Read the model definition and answer for the solid it produces. Units are mm, in the model's axes. Face numbers are marked on the shaded views. A direction names the side the tool comes from. Give positions to 0.01 mm unless a question says otherwise; leave off trailing zeros. Loops run counter-clockwise (first coordinate to the right, second up) from the corner with the lowest first, then second, coordinate; pieces in that order, holes last. Notation, with made-up numbers: (-27, -22.75) - (21, -22.75) arc R6 cw to (21, -12.75) - close; hole circle Ø1 at (65.25, -2.5). An arc over 180 degrees is marked (long way). Write each question's results on one line, items separated by ' | '. Start each with the question number.
Q1. The part is cut by section B-B, the plane x = 27.5. Write down the section's boundary in (y, z).
Q2. The part is cut by section A-A, the plane y = 10. State how many separate pieces and enclosed holes the cut face has, plus the area to 3 significant figures.
Q3. For the marked faces 1, 2 and 3, determine the directions among +Z, -Z, +X, -X, +Y, -Y from which every point of the face is accessible in a straight line to the end or side of a thin tool.
Q4. The part is cut by section D-D, the plane x = 8. Write down the section's boundary in (y, z), plus the area to 3 significant figures.
Q5. Given pin 1 (3 mm diameter, centred on x = 11.5, y = 45, fed in from -Z); pin 2 (7 mm diameter, centred on y = 51.5, z = -20, fed in from -X); pin 3 (4.5 mm diameter, centred on y = 60.5, z = 8, fed in from -X), each flat-ended and moving along its own axis, determine where each tip first touches the part or whether it passes through.
Q6. The part is cut by section C-C, the plane y = 53. Write down the section's boundary in (x, z), plus the area to 3 significant figures.
Q7. Find the intervals of material crossed by line 1 (Y direction, x = 50, z = -10); line 2 (X direction, y = 7.5, z = 18.5); line 3 (Z direction, x = 27, y = 11), in increasing order. Write a range as from..to.
Q8. Determine the mould class of the marked faces 4, 5, 6 and 7 for opening direction Z: +Z half, -Z half, draft (parallel to the pull), parting line (faces both ways), or undercut.
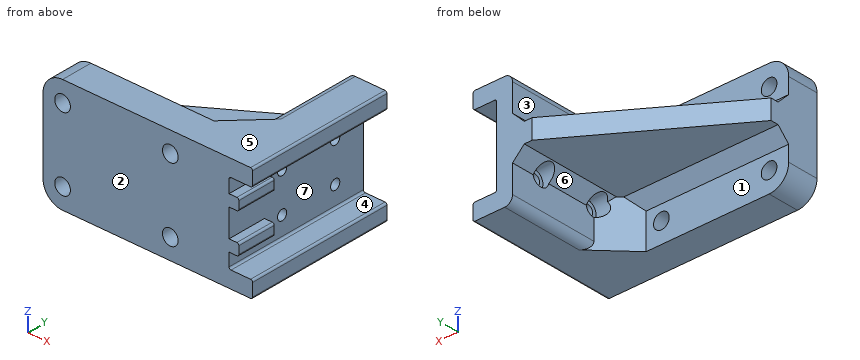
```python
from build123d import *

# Parameters (mm, degrees)
ESQUISSE1_W             = 75
ESQUISSE1_H             = 58
ESQUISSE1_R             = 4
BOSS_EXTRU_1_DEPTH      = 16
ESQUISSE2_W             = 58
ESQUISSE2_H             = 16
BOSS_EXTRU_2_DEPTH      = 20
ESQUISSE3_W             = 8.190465892
ESQUISSE3_H             = 58
BOSS_EXTRU_3_DEPTH      = 60
ESQUISSE4_W             = 8.5
ESQUISSE4_H             = 76
BOSS_EXTRU_4_DEPTH      = 12
ESQUISSE5_W             = 5.9
ESQUISSE5_H             = 20
BOSS_EXTRU_5_DEPTH      = 5
ESQUISSE6_W             = 10
ESQUISSE6_H             = 60
BOSS_EXTRU_6_DEPTH      = 86.809534108
ESQUISSE7_R             = 2.6
ENL_V_MAT_EXTRU_1_DEPTH = 119.965941395
ESQUISSE8_R             = 4.5
ENL_V_MAT_EXTRU_2_DEPTH = 3
ENL_V_MAT_EXTRU_3_DEPTH = 109.45390726
CHANFREIN1_SIZE         = 14
CHANFREIN2_SIZE         = 6
CHANFREIN3_SIZE         = 6
CONG_1_R                = 10
CONG_2_R                = 4
CONG_3_R                = 1
CONG_4_R                = 1


with BuildPart() as part:
    # Esquisse1 → Boss.-Extru.1 (new body)
    with BuildSketch(Plane(origin=(0, 0, 0), x_dir=(1, 0, 0), z_dir=(0, 1, 0))):
        Rectangle(ESQUISSE1_W, ESQUISSE1_H)
        with Locations(Location((-27.5, 18.5, 0), (0, 0, 270))):
            Circle(ESQUISSE1_R, mode=Mode.SUBTRACT)
        with Locations(Location((27.5, 18.5, 0), (0, 0, 90))):
            Circle(ESQUISSE1_R, mode=Mode.SUBTRACT)
        with Locations(Location((27.5, -18.5, 0), (0, 0, 270))):
            Circle(ESQUISSE1_R, mode=Mode.SUBTRACT)
        with Locations(Location((-27.5, -18.5, 0), (0, 0, 90))):
            Circle(ESQUISSE1_R, mode=Mode.SUBTRACT)
    extrude(amount=BOSS_EXTRU_1_DEPTH)

    # Esquisse2 → Boss.-Extru.2 (add)
    with BuildSketch(Plane(origin=(37.5, 0, 0), x_dir=(0, 0, -1), z_dir=(1, 0, 0))):
        with Locations((0, 8)):
            Rectangle(ESQUISSE2_W, ESQUISSE2_H)
    extrude(amount=BOSS_EXTRU_2_DEPTH)

    # Esquisse3 → Boss.-Extru.3 (add)
    with BuildSketch(Plane(origin=(0, 16, 0), x_dir=(1, 0, 0), z_dir=(0, 1, 0))):
        with Locations((53.404767054, 0)):
            Rectangle(ESQUISSE3_W, ESQUISSE3_H)
    extrude(amount=BOSS_EXTRU_3_DEPTH)

    # Esquisse4 → Boss.-Extru.4 (add)
    with BuildSketch(Plane(origin=(57.5, 0, 0), x_dir=(0, 0, -1), z_dir=(1, 0, 0))):
        with Locations((24.75, 38)):
            Rectangle(ESQUISSE4_W, ESQUISSE4_H)
        with Locations((-24.75, 38)):
            Rectangle(ESQUISSE4_W, ESQUISSE4_H)
    extrude(amount=BOSS_EXTRU_4_DEPTH)

    # Esquisse5 → Boss.-Extru.5 (add)
    with BuildSketch(Plane(origin=(57.5, 0, 0), x_dir=(0, 0, -1), z_dir=(1, 0, 0))):
        with Locations((-10, 10)):
            Rectangle(ESQUISSE5_W, ESQUISSE5_H)
        with Locations((10, 10)):
            Rectangle(ESQUISSE5_W, ESQUISSE5_H)
    extrude(amount=BOSS_EXTRU_5_DEPTH)

    # Esquisse6 → Boss.-Extru.6 (add)
    with BuildSketch(Plane.ZY.offset(-49.309534108)):
        with Locations((0, 46)):
            Rectangle(ESQUISSE6_W, ESQUISSE6_H)
    extrude(amount=BOSS_EXTRU_6_DEPTH)

    # Esquisse7 → Enlèv. mat.-Extru.1 (cut, through all)
    with BuildSketch(Plane.ZY.offset(-49.309534108)):
        with Locations((-10, 60)):
            Circle(ESQUISSE7_R)
        with Locations((-10, 30)):
            Circle(ESQUISSE7_R)
        with Locations(Location((10, 30, 0), (0, 0, 180))):
            Circle(ESQUISSE7_R)
        with Locations(Location((10, 60, 0), (0, 0, 180))):
            Circle(ESQUISSE7_R)
    extrude(amount=-ENL_V_MAT_EXTRU_1_DEPTH, mode=Mode.SUBTRACT)

    # Esquisse8 → Enlèv. mat.-Extru.2 (cut)
    with BuildSketch(Plane.ZY.offset(-49.309534108)):
        with Locations((-10, 60)):
            Circle(ESQUISSE8_R)
        with Locations((-10, 30)):
            Circle(ESQUISSE8_R)
        with Locations((10, 60)):
            Circle(ESQUISSE8_R)
        with Locations((10, 30)):
            Circle(ESQUISSE8_R)
    extrude(amount=-ENL_V_MAT_EXTRU_2_DEPTH, mode=Mode.SUBTRACT)

    # Esquisse9 → Enlèv. mat.-Extru.3 (cut, through all)
    with BuildSketch(Plane(origin=(0, 0, -5), x_dir=(-1, 0, 0), z_dir=(0, 0, -1))):
        Polygon((-39.309534108, 76), (37.5, 26), (37.5, 76), align=None)
    extrude(amount=-ENL_V_MAT_EXTRU_3_DEPTH, mode=Mode.SUBTRACT)

    # Chanfrein1
    # the kernel refuses this chamfer: 14 mm, written as the material it adds along each edge
    with BuildSketch(Plane(origin=(49.309534108, 16, -31.003561832), x_dir=(-0.9996219169112968, -0.027495876610586358, 0), z_dir=(0, 0, 1))) as chanfrein1_piece_1_section:
        Polygon((CHANFREIN1_SIZE * 0.999621916911, -CHANFREIN1_SIZE * 0.0274958766106), (-CHANFREIN1_SIZE * 0.0274958766106, -CHANFREIN1_SIZE * 0.999621916911), (0, 0), align=None)
    chanfrein1_piece_1 = extrude(amount=60.003561832, mode=Mode.PRIVATE)
    chanfrein1_piece_1 = split(chanfrein1_piece_1, bisect_by=Plane(origin=(44.612270729, 20.464073152, -29), z_dir=(0, 0, 1)), keep=Keep.TOP, mode=Mode.PRIVATE)
    chanfrein1_piece_1 = chanfrein1_piece_1 - Plane(origin=(44.612270729, 30, -10), x_dir=(0, 0, 1), z_dir=(-1, 0, 0)) * Cylinder(4.5, 176, mode=Mode.PRIVATE)
    chanfrein1_piece_1 = chanfrein1_piece_1 - Plane(origin=(44.612270729, 30, 10), x_dir=(0, 0, 1), z_dir=(-1, 0, 0)) * Cylinder(4.5, 176, mode=Mode.PRIVATE)
    add(chanfrein1_piece_1)
    with BuildSketch(Plane(origin=(49.309534108, 16, -29), x_dir=(0.02749587661058661, 0.9996219169112968, 0), z_dir=(0, 0, 1))) as chanfrein1_piece_2_section:
        Polygon((CHANFREIN1_SIZE * 0.999621916911, CHANFREIN1_SIZE * 0.0274958766106), (-CHANFREIN1_SIZE * 0.0274958766106, CHANFREIN1_SIZE * 0.999621916911), (0, 0), align=None)
    chanfrein1_piece_2 = extrude(amount=60.003561832, mode=Mode.PRIVATE)
    chanfrein1_piece_2 = chanfrein1_piece_2 - Plane(origin=(44.577827309, 30, -10), x_dir=(0, 0, 1), z_dir=(-1, 0, 0)) * Cylinder(4.5, 176, mode=Mode.PRIVATE)
    chanfrein1_piece_2 = split(chanfrein1_piece_2, bisect_by=Plane(origin=(44.577827309, 20.39830905, 29), z_dir=(0, 0, -1)), keep=Keep.TOP, mode=Mode.PRIVATE)
    chanfrein1_piece_2 = chanfrein1_piece_2 - Plane(origin=(44.577827309, 30, 10), x_dir=(0, 0, 1), z_dir=(-1, 0, 0)) * Cylinder(4.5, 176, mode=Mode.PRIVATE)
    add(chanfrein1_piece_2)

    # Chanfrein2
    chanfrein2_edges = [part.edges().sort_by_distance(p)[0] for p in [
        (-1.095232946, 16, 5),
        (-1.095232946, 16, -5),
    ]]
    chamfer(chanfrein2_edges, length=CHANFREIN2_SIZE)

    # Chanfrein3
    # the kernel refuses this chamfer: 6 mm, written as the material it adds along each edge
    with BuildSketch(Plane(origin=(49.309534108, 76, 5), x_dir=(-0.9996219169112968, 0, -0.027495876610586334), z_dir=(0, -1, 0))) as chanfrein3_piece_1_section:
        Polygon((CHANFREIN3_SIZE * 0.999621916911, -CHANFREIN3_SIZE * 0.0274958766106), (-CHANFREIN3_SIZE * 0.0274958766106, -CHANFREIN3_SIZE * 0.999621916911), (0, 0), align=None)
    chanfrein3_piece_1 = extrude(amount=61.430097928, mode=Mode.PRIVATE)
    chanfrein3_piece_1 = chanfrein3_piece_1 - Plane(origin=(47.194482269, 30, 10), x_dir=(0, 0, 1), z_dir=(-1, 0, 0)) * Cylinder(4.5, 147, mode=Mode.PRIVATE)
    chanfrein3_piece_1 = chanfrein3_piece_1 - Plane(origin=(47.194482269, 60, 10), x_dir=(0, 0, 1), z_dir=(-1, 0, 0)) * Cylinder(4.5, 147, mode=Mode.PRIVATE)
    add(chanfrein3_piece_1)
    with BuildSketch(Plane(origin=(49.309534108, 14.569902072, -5), x_dir=(-0.9996219169112968, 0, 0.027495876610586334), z_dir=(0, 1, 0))) as chanfrein3_piece_2_section:
        Polygon((CHANFREIN3_SIZE * 0.999621916911, -CHANFREIN3_SIZE * 0.0274958766106), (-CHANFREIN3_SIZE * 0.0274958766106, -CHANFREIN3_SIZE * 0.999621916911), (0, 0), align=None)
    chanfrein3_piece_2 = extrude(amount=61.430097928, mode=Mode.PRIVATE)
    chanfrein3_piece_2 = chanfrein3_piece_2 - Plane(origin=(47.377575529, 30, -10), x_dir=(0, 0, 1), z_dir=(-1, 0, 0)) * Cylinder(4.5, 147, mode=Mode.PRIVATE)
    chanfrein3_piece_2 = chanfrein3_piece_2 - Plane(origin=(47.377575529, 60, -10), x_dir=(0, 0, 1), z_dir=(-1, 0, 0)) * Cylinder(4.5, 147, mode=Mode.PRIVATE)
    add(chanfrein3_piece_2)

    # Congé1
    cong_1_edges = [part.edges().sort_by_distance(p)[0] for p in [
        (-37.5, 8, -29),
        (-37.5, 8, 29),
    ]]
    fillet(cong_1_edges, radius=CONG_1_R)

    # Congé2
    cong_2_edges = [part.edges().sort_by_distance(p)[0] for p in [
        (49.309534108, 53, -29),
        (49.309534108, 53, 29),
    ]]
    fillet(cong_2_edges, radius=CONG_2_R)

    # Congé3
    cong_3_edges = [part.edges().sort_by_distance(p)[0] for p in [
        (69.5, 38, 29),
        (69.5, 38, 20.5),
        (69.5, 38, -20.5),
        (69.5, 38, -29),
    ]]
    fillet(cong_3_edges, radius=CONG_3_R)

    # Congé4
    cong_4_edges = [part.edges().sort_by_distance(p)[0] for p in [
        (57.5, 38, 20.5),
        (57.5, 38, -20.5),
        (62.5, 10, 12.95),
        (62.5, 10, 7.05),
        (62.5, 10, -7.05),
        (62.5, 10, -12.95),
    ]]
    fillet(cong_4_edges, radius=CONG_4_R)


solid = part.part
```
Check sheet entries:
1) outline: (0, -29) - (16, -29) - (16, -22.5) - (0, -22.5) - close; (0, -14.5) - (16, -14.5) - (16, -11) - (22, -5) - (68.31, -5) - (68.31, 5) - (22, 5) - (16, 11) - (16, 14.5) - (0, 14.5) - close; (0, 22.5) - (16, 22.5) - (16, 29) - (0, 29) - close
2) separate pieces: 1 | enclosed holes: 4 | area: 5,530 mm^2
3) face 1: -Z, -X, +Y | face 2: +Z, -Z, +X, -X, -Y | face 3: +Z, -X, +Y
4) outline: (0, -29) - (16, -29) - (16, -11) - (22, -5) - (55.62, -5) - (55.62, 5) - (22, 5) - (16, 11) - (16, 29) - (0, 29) - close | area: 1,360 mm^2
5) pin 1: stops at z = -5 | pin 2: stops at x = 49.31 | pin 3: stops at x = 52.31
6) outline: (3.98, -5) - (43.31, -5) - (49.31, -11) - (49.31, -25) arc R4 ccw to (53.31, -29) - (68.5, -29) arc R1 ccw to (69.5, -28) - (69.5, -21.5) arc R1 ccw to (68.5, -20.5) - (58.5, -20.5) arc R1 cw to (57.5, -19.5) - (57.5, 19.5) arc R1 cw to (58.5, 20.5) - (68.5, 20.5) arc R1 ccw to (69.5, 21.5) - (69.5, 28) arc R1 ccw to (68.5, 29) - (53.31, 29) arc R4 ccw to (49.31, 25) - (49.31, 11) - (43.31, 5) - (3.98, 5) - close | area: 1,160 mm^2
7) line 1: y = 0..25.5, 34.5..55.5, 64.5..76 | line 2: x = -37.5..-31.5, -23.5..23.5, 31.5..57.5 | line 3: z = -29..-22.47, -14.53..14.53, 22.47..29
8) face 4: undercut | face 5: +Z half | face 6: -Z half | face 7: undercut
